```python
from build123d import *

# Parameters (mm, degrees)
SKETCH1_W           = 60
SKETCH1_H           = 35
SKETCH1_R           = 3.25
BOSS_EXTRUDE1_DEPTH = 1.5875
SKETCH2_R           = 2
CUT_EXTRUDE1_DEPTH  = 2.5875


with BuildPart() as part:
    # Sketch1 → Boss-Extrude1 (new body)
    with BuildSketch(Plane(origin=(0, 0, 0), x_dir=(1, 0, 0), z_dir=(0, 1, 0))):
        Rectangle(SKETCH1_W, SKETCH1_H)
        with Locations((-25.6, 12.7)):
            Circle(SKETCH1_R, mode=Mode.SUBTRACT)
        with Locations((25.2, 12.7)):
            Circle(SKETCH1_R, mode=Mode.SUBTRACT)
        with Locations((-25.6, -12.7)):
            Circle(SKETCH1_R, mode=Mode.SUBTRACT)
        with Locations((25.2, -12.7)):
            Circle(SKETCH1_R, mode=Mode.SUBTRACT)
    extrude(amount=BOSS_EXTRUDE1_DEPTH)

    # Sketch2 → Cut-Extrude1 (cut, through all)
    with BuildSketch(Plane(origin=(0, 1.5875, 0), x_dir=(1, 0, 0), z_dir=(0, 1, 0))):
        with Locations((-2.5, 10.75)):
            Circle(SKETCH2_R)
    extrude(amount=-CUT_EXTRUDE1_DEPTH, mode=Mode.SUBTRACT)


solid = part.part
```
Geometry check sheet. Reference: the model listing, model coordinates, mm. Give positions to 0.01 mm unless a question says otherwise; leave off trailing zeros. Order: outer loops, then holes, each group sorted by start corner. A loop starts at its lowest first (then second) coordinate and runs counter-clockwise, first axis right, second up.
1. Section check D-D, the plane z = -10.75. Enter the section's corners in (x, y), and give its area (3 significant figures).
2. Section check B-B, the plane x = -2.5. Enter the section's corners in (y, z).
3. Section check A-A, the plane z = 12.7. Enter the section's corners in (x, y), and give its area (3 significant figures).
4. Thickness scan on L1, parallel to Z at x = -25.6, y = 0.7; L2, parallel to X at y = 0.5, z = 12.7; L3, parallel to X at y = 0.4, z = -10.75. Record the ranges inside material, lowest first.
5. Section check C-C, the plane y = 1. Enter the section's corners in (x, z).
6. Gauge pin test, flat end, axial feed: pin 1 Ø2.5 at (x, z) = (-2.5, -10.75) entering from -Y. Record the tip position at first contact, or that the pin passes through.
7. Release check for a two-part mould opening along X. For faces 1 (the face through (24.495, 0.783, -9.527)), 2 (the face through (0, 0, 0)), 3 (the face through (30, 1, 0)) record: pulls with the +X half, pulls with the -X half, needs draft (parallel to the pull), parting line crosses it, or undercut.
Values follow:
1. outline: (-30, 0) - (-28.2, 0) - (-28.2, 1.59) - (-30, 1.59) - close; (-23, 0) - (-4.5, 0) - (-4.5, 1.59) - (-23, 1.59) - close; (-0.5, 0) - (22.6, 0) - (22.6, 1.59) - (-0.5, 1.59) - close; (27.8, 0) - (30, 0) - (30, 1.59) - (27.8, 1.59) - close
1. area: 72.4 mm2
2. outline: (0, -17.5) - (1.59, -17.5) - (1.59, -12.75) - (0, -12.75) - close; (0, -8.75) - (1.59, -8.75) - (1.59, 17.5) - (0, 17.5) - close
3. outline: (-30, 0) - (-28.85, 0) - (-28.85, 1.59) - (-30, 1.59) - close; (-22.35, 0) - (21.95, 0) - (21.95, 1.59) - (-22.35, 1.59) - close; (28.45, 0) - (30, 0) - (30, 1.59) - (28.45, 1.59) - close
3. area: 74.6 mm2
4. L1: z = -17.5 to -15.95, -9.45 to 9.45, 15.95 to 17.5
4. L2: x = -30 to -28.85, -22.35 to 21.95, 28.45 to 30
4. L3: x = -30 to -28.2, -23 to -4.5, -0.5 to 22.6, 27.8 to 30
5. outline: (-30, -17.5) - (30, -17.5) - (30, 17.5) - (-30, 17.5) - close; hole circle Ø6.5 at (-25.6, -12.7); hole circle Ø6.5 at (-25.6, 12.7); hole circle Ø4 at (-2.5, -10.75); hole circle Ø6.5 at (25.2, -12.7); hole circle Ø6.5 at (25.2, 12.7)
6. pin 1: passes through
7. face 1: undercut
7. face 2: needs draft
7. face 3: pulls with the +X half
